Verification items for the finished model (mm, model axes). Face numbers are marked on the shaded views. A direction names the side the tool comes from. Round coordinates to 2 decimals unless told otherwise and drop trailing zeros. Write each loop counter-clockwise with the first axis right and the second up, starting at its lowest first coordinate (ties: lowest second). Pieces come first, ordered by that corner, then holes. Notation, with made-up numbers: M 4.25,85.5 L 23.25,85.5 A18 ccw 23.25,112.5 Z; hole C 38.25,86.25 d11. An arc over 180 degrees is marked long. One line per item, written item: value. Start each with the question number.
Item 1: Section check C-C, the plane z = 28. Record the cut outline in (x, y), then the cut area to 3 significant figures.
Item 2: Gauge pin test, flat ends, axial feed: pin 1 (3 mm diameter, centred on x = -30, y = 7, fed in from -Z); pin 2 (2.5 mm diameter, centred on x = 23.5, z = 19, fed in from +Y); pin 3 (3.5 mm diameter, centred on x = -35.8, z = 3, fed in from +Y); pin 4 (3 mm diameter, centred on x = 15.5, z = 26.5, fed in from +Y). Record the tip position at first contact, or that the pin passes through.
Item 3: Tool access check on the marked faces 4, 5, 6 and 7. Record the directions out of +Z, -Z, +X, -X, +Y, -Y that give a thin tool (end or side, any length) a straight path to the whole face; none if there is none.
Item 4: Section check B-B, the plane y = 13. Record the cut outline in (x, z), then the cut area to 3 significant figures.
Item 5: Section check A-A, the plane z = 3. State how many separate pieces and enclosed holes the cut face has, then the cut area to 3 significant figures.
Item 6: Thickness scan on probe 1 along X at (y, z) = (16.5, 22); probe 2 along X at (y, z) = (13, 13); probe 3 along X at (y, z) = (29, 6). Record the ranges inside material, lowest first. Write a range as from..to.
Item 7: Draft check along X on the marked faces 1, 2 and 3. Enter one of: +X half, -X half, draft (parallel to the pull), parting line (faces both ways), or undercut.
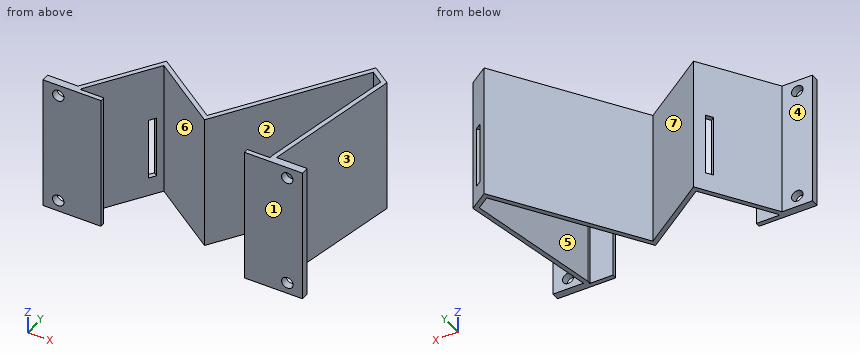
from build123d import *

# Parameters (mm, degrees)
F0_W     = 4
F0_H     = 2
F1_DEPTH = 36
F0_W_2   = 37.6
F0_H_2   = 1.2
F2_DEPTH = 36
F3_R     = 1.5
F4_DEPTH = 3
F5_W     = 2
F5_H     = 16.5
F6_DEPTH = 2
F8_DEPTH = 25


with BuildPart() as f1:
    # F0 (on Top) → F1 (new body)
    with BuildSketch(Plane.XY):
        Polygon((-39.799847, 0), (-35.799847, 0), (-31.799847, 0), (-31.799847, 2), (-39.799847, 2), align=None)
        with Locations((22.200153, 1)):
            Rectangle(F0_W, F0_H)
        with Locations((26.200153, 1)):
            Rectangle(F0_W, F0_H)
        Polygon((-31.799847, 2), (-31.799847, 0), (-24.599847, 0), (-24.599847, 1.2), (-30.599847, 1.2), (-30.599847, 1.621641), (-18.886474, 18.350071), (-0.865129, 5.731389), (23.225081, 40.135775), (26.507962, 37.837077), (19.000153, 2.124774), (19.000153, 1.2), (13.000153, 1.2), (13.000153, 0), (20.200153, 0), (20.200153, 2), (27.845302, 38.365591), (22.93039, 41.807049), (-1.15982, 7.402663), (-19.181165, 20.021345), align=None)
    extrude(amount=F1_DEPTH)

    # F0 (on Top) → F2 (cut)
    with BuildSketch(Plane.XY):
        with Locations((-5.799847, 0.6)):
            Rectangle(F0_W_2, F0_H_2)
    extrude(amount=-F2_DEPTH, mode=Mode.SUBTRACT)

    # F3 (on face) → F4 (cut)
    with BuildSketch(Plane.XZ):
        with Locations((-35.799847, 33)):
            Circle(F3_R)
        with Locations((24.200153, 33)):
            Circle(F3_R)
        with Locations((24.200153, 3)):
            Circle(F3_R)
        with Locations((-35.799847, 3)):
            Circle(F3_R)
    extrude(amount=-F4_DEPTH, mode=Mode.SUBTRACT)

    # F5 (on face) → F6 (cut)
    with BuildSketch(Plane(origin=(-22.27771, 15.599021, 0), x_dir=(-0.573576, -0.819152, 0), z_dir=(-0.819152, 0.573576, 0))):
        with Locations((-1.398661, 13.25)):
            Rectangle(F5_W, F5_H)
    extrude(amount=-F6_DEPTH, mode=Mode.SUBTRACT)

    # F7 (on face) → F8 (cut)
    with BuildSketch(Plane(origin=(26.498464, 37.843728, 0), x_dir=(0.819152, -0.573576, 0), z_dir=(-0.573576, -0.819152, 0))):
        Polygon((-2.992234, 5), (-1.992234, 5), (-0.992234, 5), (-0.992234, 21.5), (-2.992234, 21.5), align=None)
    extrude(amount=-F8_DEPTH, mode=Mode.SUBTRACT)


solid = f1.part
Response values:
1. outline: M -39.8,0 L -24.6,0 L -24.6,1.2 L -30.6,1.2 L -30.6,1.62 L -18.89,18.35 L -0.87,5.73 L 23.23,40.14 L 26.51,37.84 L 19,2.12 L 19,1.2 L 13,1.2 L 13,0 L 28.2,0 L 28.2,2 L 20.2,2 L 27.85,38.37 L 22.93,41.81 L -1.16,7.4 L -19.18,20.02 L -31.8,2 L -39.8,2 Z
1. area: 203 mm2
2. pin 1: stops at z = 0
2. pin 2: stops at y = 41.81
2. pin 3: stops at y = 2
2. pin 4: stops at y = 33.34
3. face 4: +Z, -Z, -X, +Y
3. face 5: +Z, -Z
3. face 6: +Z, -Z, -Y
3. face 7: +Z, -Z, +Y
4. outline: M -24.1,0 L -22.63,0 L -22.63,36 L -24.1,36 Z; M -11.25,0 L -9.15,0 L -9.15,36 L -11.25,36 Z; M 2.76,0 L 4.22,0 L 4.22,36 L 2.76,36 Z; M 21.29,0 L 22.51,0 L 22.51,36 L 21.29,36 Z
4. area: 225 mm2
5. separate pieces: 3
5. enclosed holes: 0
5. area: 191 mm2
6. probe 1: x = -21.65..-20.18, -16.24..-14.15, 5.21..6.68, 22.02..23.25
6. probe 2: x = -24.1..-22.63, -11.25..-9.15, 2.76..4.22, 21.29..22.51
6. probe 3: x = 13.96..15.43, 24.65..25.88
7. face 1: draft
7. face 2: undercut
7. face 3: +X half
